Source: CAD feature listing. Evaluate the final solid. Frame: model axes, mm. Face numbers are marked on the shaded views. Round coordinates to 2 decimals unless told otherwise and drop trailing zeros. Order: outer loops, then holes, each group sorted by start corner. A loop starts at its lowest first (then second) coordinate and runs counter-clockwise, first axis right, second up.
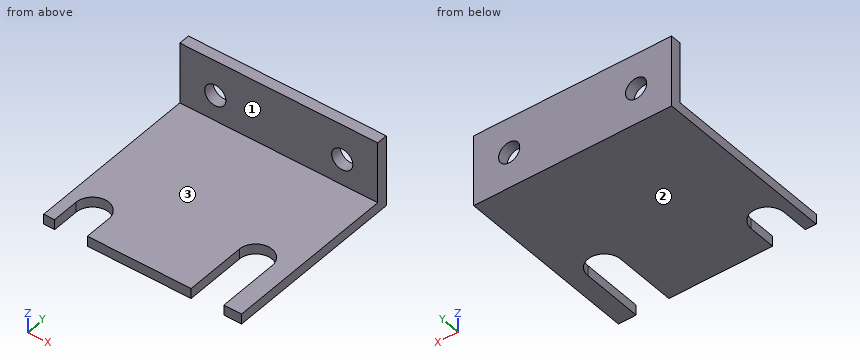
```python
from build123d import *

# Parameters (mm, degrees)
BOX_W           = 29
BOX_H           = 27
BOX_DEPTH       = 1.5
POCKET_DEPTH    = 1.501
SKETCH001_W     = 29
SKETCH001_H     = 1.6
PAD_DEPTH       = 9
SKETCH002_R     = 1.55
POCKET001_DEPTH = 27.001


with BuildPart() as part:
    # Box → Box (new body)
    with BuildSketch(Plane.XY):
        with Locations((14.5, 13.5)):
            Rectangle(BOX_W, BOX_H)
    extrude(amount=BOX_DEPTH)

    # Sketch → Pocket (cut, through all)
    with BuildSketch(Plane.XY.offset(1.5)):
        with BuildLine():
            ThreePointArc((6.399962, 4.013566), (4, 6.4), (1.600038, 4.013566))
            Line((1.600038, 4.013566), (1.600038, 0))
            Line((1.600038, 0), (6.399962, 0))
            Line((6.399962, 4.013566), (6.399962, 0))
        make_face()
        with BuildLine():
            Line((21.6, 8.999953), (21.6, 0))
            Line((21.6, 0), (26.4, 0))
            Line((26.4, 8.999953), (26.4, 0))
            ThreePointArc((26.4, 8.999953), (24, 11.4), (21.6, 8.999953))
        make_face()
    extrude(amount=-POCKET_DEPTH, mode=Mode.SUBTRACT)

    # Sketch001 → Pad (new body)
    with BuildSketch(Plane.XY.offset(1.5)):
        with Locations((14.5, 26.2)):
            Rectangle(SKETCH001_W, SKETCH001_H)
    extrude(amount=PAD_DEPTH)

    # Sketch002 → Pocket001 (cut, through all)
    with BuildSketch(Plane(origin=(0, 27, 0), x_dir=(-1, 0, 0), z_dir=(0, 1, 0))):
        with Locations((-23.8, 5.31)):
            Circle(SKETCH002_R)
        with Locations((-5.2, 5.31)):
            Circle(SKETCH002_R)
    extrude(amount=-POCKET001_DEPTH, mode=Mode.SUBTRACT)


solid = part.part
```
1. Line query: line 1 along Z through (x, y) = (5.2, 26.6); line 2 along Z through (x, y) = (3.5, 20.5); line 3 along Y through (x, z) = (20.75, 4.75). Output: solid intervals per line, ascending.
2. Pull-direction query (Z, two-part tool) for the marked faces 1, 2 and 3; classes: released by +Z, released by -Z, zero draft, split by the parting line, or undercut.
3. Section A-A on y = 7.25. Return loops of the section in (x, z), plus the area to 3 significant figures.
4. First-contact query: pin 1 (5 mm diameter, centred on x = 5.2, z = 5.31, fed in from +Y); pin 2 (4.5 mm diameter, centred on x = 19.5, z = 4, fed in from -Y); pin 3 (12.5 mm diameter, centred on x = 16, y = 13.5, fed in from +Z). Flat tips, straight axial feed; report the tip coordinate or a pass-through.
5. Section D-D on z = 4.75. Return loops of the section in (x, y).
6. Section C-C on y = 2. Return loops of the section in (x, z), plus the area to 3 significant figures.
7. Section B-B on x = 5.2. Return loops of the section in (y, z), plus the area to 3 significant figures.
Result:
1. line 1: z = 0 to 3.76, 6.86 to 10.5
1. line 2: z = 0 to 1.5
1. line 3: y = 25.4 to 27
2. face 1: zero draft
2. face 2: released by -Z
2. face 3: released by +Z
3. outline: (0, 0) - (21.6, 0) - (21.6, 1.5) - (0, 1.5) - close; (26.4, 0) - (29, 0) - (29, 1.5) - (26.4, 1.5) - close
3. area: 36.3 mm2
4. pin 1: stops at y = 27
4. pin 2: stops at y = 25.4
4. pin 3: stops at z = 1.5
5. outline: (0, 25.4) - (3.75, 25.4) - (3.75, 27) - (0, 27) - close; (6.65, 25.4) - (22.35, 25.4) - (22.35, 27) - (6.65, 27) - close; (25.25, 25.4) - (29, 25.4) - (29, 27) - (25.25, 27) - close
6. outline: (0, 0) - (1.6, 0) - (1.6, 1.5) - (0, 1.5) - close; (6.4, 0) - (21.6, 0) - (21.6, 1.5) - (6.4, 1.5) - close; (26.4, 0) - (29, 0) - (29, 1.5) - (26.4, 1.5) - close
6. area: 29.1 mm2
7. outline: (6.08, 0) - (27, 0) - (27, 3.76) - (25.4, 3.76) - (25.4, 1.5) - (6.08, 1.5) - close; (25.4, 6.86) - (27, 6.86) - (27, 10.5) - (25.4, 10.5) - close
7. area: 40.8 mm2
